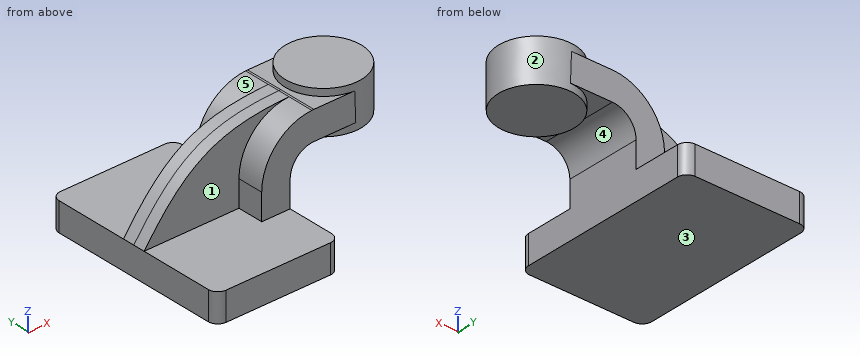
```python
from build123d import *

# Parameters (mm, degrees)
F1_DEPTH = 63.5
F0_W     = 25.3649728298
F0_H     = 19.05
F2_DEPTH = 25.4
F3_DEPTH = 7.9375
F5_R     = 6.35


with BuildPart() as f1:
    # F0 (on Front) → F1 (new body, symmetric)
    with BuildSketch(Plane.XZ):
        Polygon((-41.275, -9.525), (41.275, -9.525), (41.275, 9.525), (22.225, 9.525), (-41.275, 9.525), align=None)
    extrude(amount=F1_DEPTH, both=True)

    # F0 (on Front) → F2 (join, symmetric)
    with BuildSketch(Plane.XZ):
        with BuildLine():
            Line((22.225, 9.525), (41.275, 9.525))
            Line((41.275, 9.525), (41.275, 27.0002))
            ThreePointArc((41.275, 27.0002), (45.9246798487, 38.2255201513), (57.15, 42.8752))
            Line((57.15, 42.8752), (60.3600271702, 42.8752))
            Line((60.3600271702, 42.8752), (60.3600271702, 61.9252))
            Line((60.3600271702, 61.9252), (57.15, 61.9252))
            add(Edge.make_bspline(
                [(55.8049149759, 61.8992884018), (56.250937163, 61.9088103387), (56.6992894846, 61.9174422694), (57.15, 61.9252)],
                knots=[110.4669042638, 110.4669042638, 110.4669042638, 110.4669042638, 111.5045361635, 111.5045361635, 111.5045361635, 111.5045361635], degree=3))
            ThreePointArc((55.8049149759, 61.8992884018), (31.9832290563, 51.215675739), (22.225, 27.0002))
            Line((22.225, 27.0002), (22.225, 9.525))
        make_face()
        with Locations((73.0425135851, 52.4002)):
            Rectangle(F0_W, F0_H)
    extrude(amount=F2_DEPTH, both=True)

    # F0 (on Front) → F3 (join, symmetric)
    with BuildSketch(Plane.XZ):
        with BuildLine():
            add(Edge.make_bspline(
                [(-41.275, 9.525), (-12.7532446295, 49.7846645012), (8.3211297732, 60.8855773876), (55.8049149759, 61.8992884018)],
                knots=[0, 0, 0, 0, 110.4669042638, 110.4669042638, 110.4669042638, 110.4669042638], degree=3))
            Line((-41.275, 9.525), (22.225, 9.525))
            Line((22.225, 9.525), (22.225, 27.0002))
            ThreePointArc((22.225, 27.0002), (31.9832290563, 51.215675739), (55.8049149759, 61.8992884018))
        make_face()
    extrude(amount=F3_DEPTH, both=True)

    # F0 (on Front) → F4 (revolve)
    with BuildSketch(Plane.XZ):
        Polygon((85.725, 66.675), (85.7600271702, 38.1), (111.1600271702, 38.1), (111.1600271702, 66.675), align=None)
    revolve(axis=Axis((85.7425135851, 0, 52.3875), (-0.0012257968, 0, 0.9999992487)))

    # F5
    f5_edges = [f1.edges().sort_by_distance(p)[0] for p in [
        (-41.275, -63.5, 0),
        (41.275, -63.5, 0),
        (41.275, 63.5, 0),
        (-41.275, 63.5, 0),
    ]]
    fillet(f5_edges, radius=F5_R)


solid = f1.part
```
The listing builds one solid part. Answer for the finished solid, in the listing's coordinates (mm). Face numbers are marked on the shaded views. A direction names the side the tool comes from. Give positions to 0.01 mm unless a question says otherwise; leave off trailing zeros. Loops run counter-clockwise (first coordinate to the right, second up) from the corner with the lowest first, then second, coordinate; pieces in that order, holes last. Notation, with made-up numbers: (-8.75, 88) - (13.25, 88) arc R27 ccw to (13.25, 109) - close; hole circle Ø5 at (44.5, 29.25). An arc over 180 degrees is marked (long way). Answer as CSV lines item,"result". Start each with the question number.
Item 1: Each of these flat-tipped pins is pushed along its axis until it touches: pin 1 (2 mm diameter, centred on y = -46, z = -1, fed in from +X) (3 decimals); pin 2 (5 mm diameter, centred on y = 14, z = 15, fed in from -X) (3 decimals); pin 3 (1.5 mm diameter, centred on x = 10.5, y = -48.5, fed in from +Z) (3 decimals). Where does it stop, or does it pass through?
Item 2: The mould has two halves that part along X. Classify the marked faces 3, 4 and 5: +X half, -X half, draft (parallel to the pull), parting line (faces both ways), or undercut.
Item 3: For the marked faces 1 and 2, determine the directions among +Z, -Z, +X, -X, +Y, -Y from which every point of the face is accessible in a straight line to the end or side of a thin tool.
Item 4: A cutting plane is placed at B-B on y = -39. Determine the outline of the cut face in (x, z) (3 decimals), then the cut area to 3 significant figures.
Item 5: Find the intervals of material crossed by line 1 (Y direction, x = -13, z = 33.5); line 2 (Z direction, x = 20.5, y = 47) (3 decimals); line 3 (Z direction, x = 88, y = -4), in increasing order. Write a range as from..to.
Item 6: A cutting plane is placed at A-A on z = 7. Determine the outline of the cut face in (x, y) (3 decimals).
Found:
1,pin 1,"stops at x = 41.275"
1,pin 2,"stops at x = 22.225"
1,pin 3,"stops at z = 9.525"
2,face 3,"draft"
2,face 4,"undercut"
2,face 5,"-X half"
3,face 1,"+Z, -X, -Y"
3,face 2,"none"
4,outline,"(-41.275, -9.525) - (41.275, -9.525) - (41.275, 9.525) - (-41.275, 9.525) - close"
4,area,"1,570 mm^2"
5,line 1,"y = -7.94..7.94"
5,line 2,"z = -9.525..9.525"
5,line 3,"z = 38.1..66.67"
6,outline,"(-41.275, -57.15) arc R6.35 ccw to (-34.925, -63.5) - (34.925, -63.5) arc R6.35 ccw to (41.275, -57.15) - (41.275, 57.15) arc R6.35 ccw to (34.925, 63.5) - (-34.925, 63.5) arc R6.35 ccw to (-41.275, 57.15) - close"
